```python
from build123d import *

# Parameters (mm, degrees)
SKETCH1_W           = 52
SKETCH1_H           = 17
BOSS_EXTRUDE1_DEPTH = 11
SKETCH2_R           = 1
BOSS_EXTRUDE2_DEPTH = 11
SKETCH3_R           = 1
SKETCH3_R_2         = 0.5
BOSS_EXTRUDE3_DEPTH = 11


with BuildPart() as part:
    # Sketch1 → Boss-Extrude1 (new body)
    with BuildSketch(Plane(origin=(0, 0, 0), x_dir=(1, 0, 0), z_dir=(0, 1, 0))):
        with Locations((26, 8.5)):
            Rectangle(SKETCH1_W, SKETCH1_H)
    extrude(amount=BOSS_EXTRUDE1_DEPTH)

    # Sketch2 → Boss-Extrude2 (add)
    with BuildSketch(Plane.ZY):
        with Locations(Location((-13, 5, 0), (0, 0, 180))):
            Circle(SKETCH2_R)
        with Locations(Location((-10.9, 5, 0), (0, 0, 180))):
            Circle(SKETCH2_R)
        with Locations(Location((-8.8, 5, 0), (0, 0, 180))):
            Circle(SKETCH2_R)
    extrude(amount=BOSS_EXTRUDE2_DEPTH)

    # Sketch3 → Boss-Extrude3 (add)
    with BuildSketch(Plane(origin=(52, 0, 0), x_dir=(0, 0, -1), z_dir=(1, 0, 0))):
        with Locations(Location((14.5, 8.5, 0), (0, 0, 180))):
            Circle(SKETCH3_R)
        with Locations(Location((14.5, 2.5, 0), (0, 0, 180))):
            Circle(SKETCH3_R)
        with Locations(Location((13.5, 6.6, 0), (0, 0, 180))):
            Circle(SKETCH3_R_2)
        with Locations(Location((13.5, 5.5, 0), (0, 0, 180))):
            Circle(SKETCH3_R_2)
        with Locations(Location((13.5, 4.4, 0), (0, 0, 180))):
            Circle(SKETCH3_R_2)
    extrude(amount=BOSS_EXTRUDE3_DEPTH)


solid = part.part
```
Geometry: final body of the model. Coordinates: model frame, mm. A direction names the side the tool comes from. Coordinates: 2 decimals unless noted, no trailing zeros. Order: outer loops, then holes, each group sorted by start corner. A loop starts at its lowest first (then second) coordinate and runs counter-clockwise, first axis right, second up. Notation, with made-up numbers: (45.5, -18.5) -> (68.5, -18.5) arc R5 cw to (68.5, -13.5) -> close; hole circle Ø6 at (-20.5, 52). An arc over 180 degrees is marked (long way). Write each question's results on one line, items separated by ' | '. Start each with the question number.
1) Cut plane B-B, the plane y = 10.25. Output: boundary loops of the cut face in (x, z), and give its area (3 significant figures).
2) Set-up query: faces 1 (the cylindrical face through (57.423, 8.2, -13.546)), 2 (the flat face through (63, 2, -15)), 3 (the cylindrical face through (-5, 4, -13)). Return all of +Z, -Z, +X, -X, +Y, -Y with unobstructed straight access to the full face (end or side cutting, diameter ignored); none if empty.
3) First-contact query: pin 1 (2 mm diameter, centred on x = 55.5, y = 8.5, fed in from +Z). Flat tip, straight axial feed; report the tip coordinate or a pass-through.
4) Material intervals for line 1 along X through (y, z) = (0.5, -16.25); line 2 along X through (y, z) = (5, -8); line 3 along Y through (x, z) = (57, -15), sorted ascending.
5) Cut plane A-A, the plane z = -8.8. Output: boundary loops of the cut face in (x, y), and give its area (3 significant figures).
6) Mould query, pull axis Z, two halves, no side actions, for faces 4 (the flat face through (26, 5, 0)), 5 (the cylindrical face through (-5.423, 4.324, -10.163)), 6 (the flat face through (26, 11, -9)). Classes: released by +Z, released by -Z, zero draft, split by the parting line, or undercut.
Checks:
1) outline: (0, -17) -> (52, -17) -> (52, 0) -> (0, 0) -> close | area: 884 mm^2
2) face 1: +X | face 2: +Z, -Z, +X, +Y, -Y | face 3: -X
3) pin 1: z = -13.5
4) line 1: 0 to 52 | line 2: -11 to 52 | line 3: 1.63 to 3.37, 7.63 to 9.37
5) outline: (-11, 4) -> (0, 4) -> (0, 0) -> (52, 0) -> (52, 11) -> (0, 11) -> (0, 6) -> (-11, 6) -> close | area: 594 mm^2
6) face 4: released by +Z | face 5: undercut | face 6: zero draft
